Build history of the part. All positions in model axes, mm. A direction names the side the tool comes from. Round coordinates to 2 decimals unless told otherwise and drop trailing zeros. Write each loop counter-clockwise with the first axis right and the second up, starting at its lowest first coordinate (ties: lowest second). Pieces come first, ordered by that corner, then holes. Notation, with made-up numbers: (-23.5, 70) - (8.5, 70) arc R25 ccw to (8.5, 103) - close; hole circle Ø4 at (12.25, 7.25). An arc over 180 degrees is marked (long way). One line per question, with ' | ' between items.
from build123d import *

# Parameters (mm, degrees)
SKETCH1_R                = 7.5
SKETCH1_R_2              = 1.5
BOSS_EXTRUDE1_DEPTH      = 2
SKETCH2_R                = 10.5
SKETCH2_R_2              = 7.5
BOSS_EXTRUDE2_DEPTH      = 7.5
BOSS_EXTRUDE4_DEPTH      = 0.5
BOSS_EXTRUDE4_DEPTH_BACK = 0.5
BOSS_EXTRUDE5_DEPTH      = 0.5
BOSS_EXTRUDE5_DEPTH_BACK = 0.5


with BuildPart() as part:
    # Sketch1 → Boss-Extrude1 (new body)
    with BuildSketch(Plane(origin=(0, 0, 0), x_dir=(1, 0, 0), z_dir=(0, 1, 0))):
        Polygon((-14.387647793, 11), (-10.387647793, 15), (10.387647793, 15), (14.387647793, 11), (14.387647793, -11), (10.387647793, -15), (-10.387647793, -15), (-14.387647793, -11), align=None)
        with Locations(Location((0, 0, 0), (0, 0, 270))):
            Circle(SKETCH1_R, mode=Mode.SUBTRACT)
        with Locations(Location((-10.69839003, -11.153723858, 0), (0, 0, 270))):
            Circle(SKETCH1_R_2, mode=Mode.SUBTRACT)
        with Locations(Location((-10.69839003, 11.153723858, 0), (0, 0, 270))):
            Circle(SKETCH1_R_2, mode=Mode.SUBTRACT)
        with Locations(Location((10.69839003, 11.153723858, 0), (0, 0, 270))):
            Circle(SKETCH1_R_2, mode=Mode.SUBTRACT)
        with Locations(Location((10.69839003, -11.153723858, 0), (0, 0, 270))):
            Circle(SKETCH1_R_2, mode=Mode.SUBTRACT)
    extrude(amount=BOSS_EXTRUDE1_DEPTH)

    # Sketch2 → Boss-Extrude2 (add)
    with BuildSketch(Plane(origin=(0, 2, 0), x_dir=(1, 0, 0), z_dir=(0, 1, 0))):
        with Locations(Location((0, 0, 0), (0, 0, 90))):
            Circle(SKETCH2_R)
        with Locations(Location((0, 0, 0), (0, 0, 270))):
            Circle(SKETCH2_R_2, mode=Mode.SUBTRACT)
    extrude(amount=BOSS_EXTRUDE2_DEPTH)

    # Sketch4 → Boss-Extrude4 (add, two sides: drawn at the far end of the back side and taken through both)
    with BuildSketch(Plane(origin=(0, 0, 0), x_dir=(0, 0, -1), z_dir=(1, 0, 0)).offset(-BOSS_EXTRUDE4_DEPTH_BACK)):
        Polygon((10.5, 9.5), (14, 2), (7.5, 2), (7.5, 9.5), align=None)
        Polygon((-10.5, 9.5), (-7.5, 9.5), (-7.5, 2), (-14, 2), align=None)
    extrude(amount=BOSS_EXTRUDE4_DEPTH + BOSS_EXTRUDE4_DEPTH_BACK)

    # Sketch5 → Boss-Extrude5 (add, two sides: drawn at the far end of the back side and taken through both)
    with BuildSketch(Plane.XY.offset(-BOSS_EXTRUDE5_DEPTH_BACK)):
        Polygon((-10.5, 9.5), (-13.387647793, 2), (-7.5, 2), (-7.5, 9.5), align=None)
        Polygon((10.5, 9.5), (13.387647793, 2), (7.5, 2), (7.5, 9.5), align=None)
    extrude(amount=BOSS_EXTRUDE5_DEPTH + BOSS_EXTRUDE5_DEPTH_BACK)


solid = part.part
Q1. Drill centre lines: L1, parallel to Y at x = 2.25, z = 11.25; L2, parallel to X at y = 5, z = 0; L3, parallel to Z at x = -9.75, y = 1.25. Where is each one in solid material? Low to high. Write a range as from..to.
Found:
L1: 0..2 | L2: -12.23..-7.5, 7.5..12.23 | L3: -15..-12.32, -9.99..9.99, 12.32..15
Q2. Pull direction X, two halves, no side cores. Call faces 5 (the flat face through (-14.388, 1, 0)), 6 (the cylindrical face through (-11.27, 0.99, 12.54)), 7 (the flat face through (12.42, 0.99, 12.97)): +X half, -X half, draft (parallel to the pull), parting line (faces both ways), or undercut.
Found:
face 5: -X half | face 6: undercut | face 7: +X half
Q3. Saw through at D-D, the plane z = -8. List the corners of the cut face in (x, y).
Found:
outline: (-14.39, 0) - (14.39, 0) - (14.39, 2) - (6.8, 2) - (6.8, 9.5) - (-6.8, 9.5) - (-6.8, 2) - (-14.39, 2) - close
Q4. Drop flat-ended pins along their axis: pin 1 (1.8 mm diameter, centred on y = 4.5, z = 12.5, fed in from +X); pin 2 (1 mm diameter, centred on y = 5.5, z = 1.5, fed in from +X); pin 3 (1.4 mm diameter, centred on x = 12.5, y = 4, fed in from +Z). Give the stop position or say it passes through.
Found:
pin 1: x = 0.5 | pin 2: x = 10.45 | pin 3: z = 0.5
Q5. Saw through at A-A, the plane x = 0. List the corners of the cut face in (y, z), then the cut area to 3 significant figures.
Found:
outline: (0, -15) - (2, -15) - (2, -14) - (9.5, -10.5) - (9.5, -7.5) - (0, -7.5) - close; (0, 7.5) - (9.5, 7.5) - (9.5, 10.5) - (2, 14) - (2, 15) - (0, 15) - close | area: 101 mm^2
Q6. Saw through at C-C, the plane y = 4.25. List the corners of the cut face in (x, z).
Found:
outline: (-12.52, -0.5) - (-10.49, -0.5) arc R10.5 ccw to (-0.5, -10.49) - (-0.5, -12.95) - (0.5, -12.95) - (0.5, -10.49) arc R10.5 ccw to (10.49, -0.5) - (12.52, -0.5) - (12.52, 0.5) - (10.49, 0.5) arc R10.5 ccw to (0.5, 10.49) - (0.5, 12.95) - (-0.5, 12.95) - (-0.5, 10.49) arc R10.5 ccw to (-10.49, 0.5) - (-12.52, 0.5) - close; hole circle Ø15 at (0, 0)
Q7. Which spindle directions (+Z, -Z, +X, -X, +Y, -Y) get a long thin tool onto all of the face, cutting with end or side? Do faces 1 (the cylindrical face through (-7.35, 5.7, -7.5)), 2 (the flat face through (0.5, 4, -11)), 3 (the cylindrical face through (7.35, 5.7, 7.5)), 4 (the flat face through (-0.5, 5, 12)). Say none if no direction does.
Found:
face 1: -Z, -X, +Y | face 2: -Z, +X, +Y | face 3: +Z, +X, +Y | face 4: +Z, -X, +Y
Q8. Saw through at B-B, the plane z = 0. List the corners of the cut face in (x, y).
Found:
outline: (-14.39, 0) - (-7.5, 0) - (-7.5, 9.5) - (-10.5, 9.5) - (-13.39, 2) - (-14.39, 2) - close; (7.5, 0) - (14.39, 0) - (14.39, 2) - (13.39, 2) - (10.5, 9.5) - (7.5, 9.5) - close
